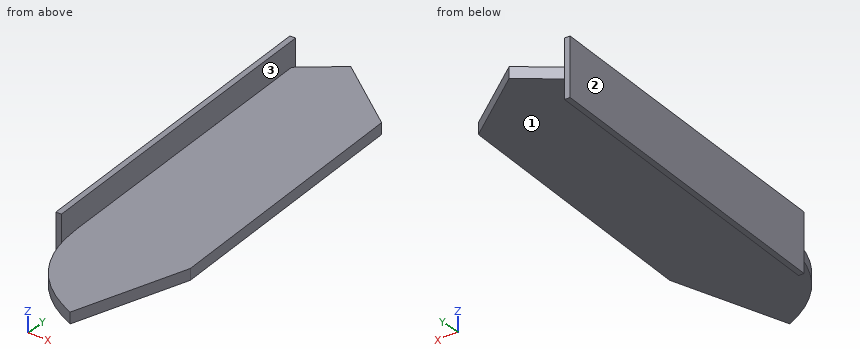
from build123d import *

# Parameters (mm, degrees)
EXTRUDE_1_DEPTH     = 1.2
CUT_EXTRUDE_START   = -1.2
CUT_EXTRUDE_1_DEPTH = 1.2
SKETCH_3_R          = 0.3
EXTRUDE_2_DEPTH     = 0.3
SKETCH_4_W          = 6.240890377
SKETCH_4_H          = 36.021981299
EXTRUDE_3_DEPTH     = 0.6


# Read off the part's stored shape, not the designer's step: Вырез-Вытянуть-Тонкостенный1
with BuildPart() as part:
    # Эскиз1 → Бобышка-Вытянуть1 (new body)
    with BuildSketch(Plane.XY):
        with BuildLine():
            Line((5.378881308, 18.237319105), (-2.952136628, 24.369097407))
            Line((-2.952136628, 24.369097407), (-7.332317287, 20.785313231))
            Line((-7.332317287, 20.785313231), (-5.370009146, -12.399066019))
            add(Edge.make_bspline(
                [(-5.370009146, -12.399066019), (-5.302441643, -13.087933403), (-5.171652717, -14.4213588), (-4.705894041, -16.337224351), (-3.980118415, -18.073869331), (-3.037863831, -19.656891462), (-1.854751161, -21.069611208), (-0.442865037, -22.322015124), (1.210414163, -23.402243504), (2.432125444, -23.961998582), (3.062087221, -24.250630037)],
                knots=[0, 0, 0, 0, 0.134544415, 0.260434655, 0.381864625, 0.499402401, 0.617479097, 0.738843694, 0.865337667, 1, 1, 1, 1], degree=3))
            Line((3.062087221, -24.250630037), (3.44414449, -24.369097407))
            Line((3.44414449, -24.369097407), (7.332317287, -11.660532618))
            Line((7.332317287, -11.660532618), (5.378881308, 18.237319105))
        make_face()
    extrude(amount=EXTRUDE_1_DEPTH)

    # Вырез-Вытянуть-Тонкостенный1 outline → Вырез-Вытянуть-Тонкостенный1 (cut)
    with BuildSketch(Plane.XY.offset(1.2).offset(CUT_EXTRUDE_START)):
        with BuildLine():
            Line((-7.332317287, 20.785313231), (-5.370009146, -12.399066019))
            add(Edge.make_bspline(
                [(-5.370009146, -12.399066019), (-5.302441643, -13.087933403), (-5.171652717, -14.4213588), (-4.705894041, -16.337224351), (-3.980118415, -18.073869331), (-3.037863831, -19.656891462), (-1.854751161, -21.069611208), (-0.442865037, -22.322015124), (1.210414163, -23.402243504), (2.432125444, -23.961998582), (3.062087221, -24.250630037)],
                knots=[0, 0, 0, 0, 0.134544415, 0.260434655, 0.381864625, 0.499402401, 0.617479097, 0.738843694, 0.865337667, 1, 1, 1, 1], degree=3))
            Line((3.062087221, -24.250630037), (3.44414449, -24.369097407))
            Line((3.44414449, -24.369097407), (7.332317287, -11.660532618))
            Line((7.332317287, -11.660532618), (5.378881308, 18.237319105))
            Line((5.378881308, 18.237319105), (-2.952136628, 24.369097407))
            Line((-2.952136628, 24.369097407), (-7.332317287, 20.785313231))
        make_face()
        with BuildLine():
            add(Edge.make_bspline(
                [(-4.971163716, -12.367724843), (-4.910437592, -12.986836229), (-4.849676357, -13.605939574), (-4.654543085, -14.827292297), (-4.518019632, -15.429049084), (-4.24283568, -16.315565722), (-4.139152476, -16.608333995), (-3.907848144, -17.188389699), (-3.77968372, -17.476760574), (-3.366686296, -18.319539943), (-3.053087929, -18.855873767), (-2.517467922, -19.616879364), (-2.327928668, -19.863212785), (-1.927678486, -20.341760794), (-1.716167659, -20.574779068), (-1.056114397, -21.24716639), (-0.586382585, -21.656301106), (0.408094083, -22.402093404), (0.932873325, -22.738705687), (2.037021143, -23.34001134), (2.608653164, -23.602856812), (3.180150897, -23.864736725)],
                knots=[0, 0, 0, 0, 0.125, 0.125, 0.25, 0.25, 0.3125, 0.3125, 0.375, 0.375, 0.5, 0.5, 0.5625, 0.5625, 0.625, 0.625, 0.75, 0.75, 0.875, 0.875, 1, 1, 1, 1], degree=3))
            Line((-4.971163716, -12.367724843), (-6.920959218, 20.605054546))
            Line((-6.920959218, 20.605054546), (-2.939165367, 23.862885878))
            Line((-2.939165367, 23.862885878), (4.991867828, 18.025503503))
            Line((4.991867828, 18.025503503), (6.928393761, -11.61353551))
            Line((6.928393761, -11.61353551), (3.180150897, -23.864736725))
        make_face(mode=Mode.SUBTRACT)
    extrude(amount=CUT_EXTRUDE_1_DEPTH, mode=Mode.SUBTRACT)

    # Эскиз3 → Бобышка-Вытянуть2 (add)
    with BuildSketch(Plane(origin=(-5.682639561, -0.336034307, 0), x_dir=(0, 0, 1), z_dir=(-0.9982561871654927, -0.059030371723486505, 0))):
        with Locations(Location((0.6, 20.377669982, 0), (0, 0, 270))):
            Circle(SKETCH_3_R)
        with Locations(Location((0.6, 9.777669982, 0), (0, 0, 270))):
            Circle(SKETCH_3_R)
        with Locations(Location((0.6, -0.822330018, 0), (0, 0, 270))):
            Circle(SKETCH_3_R)
        with Locations(Location((0.6, -11.422330018, 0), (0, 0, 270))):
            Circle(SKETCH_3_R)
    extrude(amount=EXTRUDE_2_DEPTH)

    # Эскиз4 → Бобышка-Вытянуть3 (add)
    with BuildSketch(Plane(origin=(-5.982116417, -0.353743418, 0), x_dir=(0, 0, 1), z_dir=(-0.9982561871654927, -0.05903037172348652, 0))):
        with Locations((0.435766043, 4.003532813)):
            Rectangle(SKETCH_4_W, SKETCH_4_H)
    extrude(amount=EXTRUDE_3_DEPTH)


solid = part.part
Work out the finished part from the listing and answer in its coordinate system (mm). Face numbers are marked on the shaded views. Round coordinates to 2 decimals unless told otherwise and drop trailing zeros. Order: outer loops, then holes, each group sorted by start corner. A loop starts at its lowest first (then second) coordinate and runs counter-clockwise, first axis right, second up. Notation, with made-up numbers: M -13,62.25 L 12,62.25 A13 ccw 12,73.25 Z; hole C 38,-36 d4. An arc over 180 degrees is marked long. One line per item, written item: value.
Q1. Straight lines are drawn through the part: line 1 (Z direction, x = 3.25, y = 0); line 2 (X direction, y = 11, z = 0.5); line 3 (X direction, y = 20, z = -1.5). For each, find the intervals that lie inside material, in ascending order.
Derived:
line 1: 0 to 1.2
line 2: -7.25 to -6.65, -6.35 to 5.45
line 3: -7.79 to -7.19
Q2. Find section C-C on z = -1.25. Write down the section's boundary in (x, y).
Derived:
outline: M -7.88,21.59 L -5.75,-14.37 L -5.16,-14.34 L -7.28,21.62 Z
Q3. Find section B-B on y = 4. Write down the section's boundary in (x, z).
Derived:
outline: M -6.84,-2.68 L -6.24,-2.68 L -6.24,3.56 L -6.84,3.56 Z; M -5.94,0 L 5.91,0 L 5.91,1.2 L -5.94,1.2 Z
Q4. Find section D-D on x = 5.5. Write down the section's boundary in (y, z), then the cut area to 3 significant figures.
Derived:
outline: M -16.28,0 L 10.25,0 L 10.25,1.2 L -16.28,1.2 Z
area: 31.8 mm²
Q5. Determine the mould class of the marked faces 1, 2 and 3 for opening direction X: released by +X, released by -X, zero draft, split by the parting line, or undercut.
Derived:
face 1: zero draft
face 2: released by -X
face 3: undercut
Q6. Flat-ended cylindrical pins translate along their axes: pin 1 (1 mm diameter, centred on x = -1.5, y = -17.5, fed in from -Z); pin 2 (1.5 mm diameter, centred on x = -3.5, z = -1.5, fed in from -Y); pin 3 (3 mm diameter, centred on x = -1, y = 18.5, fed in from +Z). Find the tip coordinate at first contact, or state that the pin passes through.
Derived:
pin 1: z = 0
pin 2: through
pin 3: z = 1.2
Q7. Find section A-A on y = -7.5. Write down the section's boundary in (x, z).
Derived:
outline: M -6.16,-2.68 L -5.56,-2.68 L -5.56,3.56 L -6.16,3.56 Z; M -5.26,0 L 6.66,0 L 6.66,1.2 L -5.26,1.2 Z
